from build123d import *

# Parameters (mm, degrees)
MODEL_W                 = 52
MODEL_H                 = 52
MODEL_R                 = 1.5
SALIENTE_EXTRUIR1_DEPTH = 3


with BuildPart() as part:
    # Model → Saliente-Extruir1 (new body)
    with BuildSketch(Plane.XY):
        with Locations((66, 205)):
            Rectangle(MODEL_W, MODEL_H)
        with Locations((51, 190)):
            Circle(MODEL_R, mode=Mode.SUBTRACT)
        with Locations((81, 190)):
            Circle(MODEL_R, mode=Mode.SUBTRACT)
        with Locations((81, 220)):
            Circle(MODEL_R, mode=Mode.SUBTRACT)
        with Locations((51, 220)):
            Circle(MODEL_R, mode=Mode.SUBTRACT)
        Polygon((56, 226), (56, 215), (46, 215), (46, 195), (56, 195), (56, 184), (69.4, 184), (69.4, 226), align=None, mode=Mode.SUBTRACT)
        Polygon((72.4, 226), (72.4, 184), (76, 184), (76, 195), (85, 195), (85, 215), (76, 215), (76, 226), align=None, mode=Mode.SUBTRACT)
    extrude(amount=SALIENTE_EXTRUIR1_DEPTH)


solid = part.part
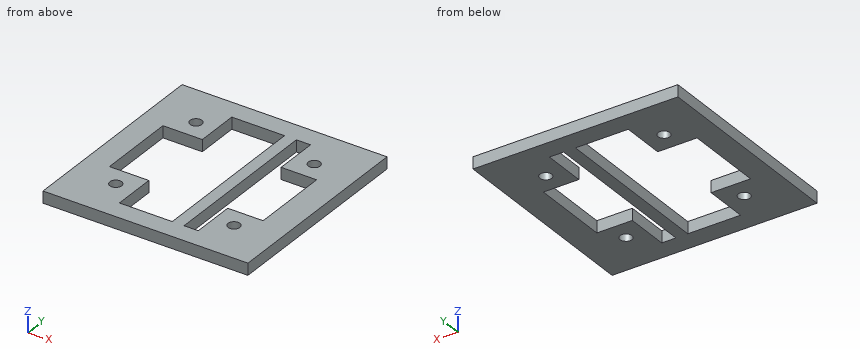
Geometry: final body of the model. Coordinates: model frame, mm. Coordinates: 2 decimals unless noted, no trailing zeros. Loops run counter-clockwise (first coordinate to the right, second up) from the corner with the lowest first, then second, coordinate; pieces in that order, holes last. Notation, with made-up numbers: M 65.5,21.5 L 117.5,21.5 A22 cw 117.5,51.5 Z; hole C 76,2.5 d11. An arc over 180 degrees is marked long. One line per item, written item: value. Start each with the question number.
1) Pin query (flat end, axial travel): P1, Ø12, axis at x = 63.5, y = 201, coming from the +Z side. Return the tip coordinate at first contact, or that it passes through.
2) Cut plane B-B (x = 51). Return loops of the section in (y, z), then the cut area to 3 significant figures.
3) Cut plane D-D (x = 77). Return loops of the section in (y, z), then the cut area to 3 significant figures.
4) Cut plane C-C (y = 190). Return loops of the section in (x, z).
5) Material intervals for L1, parallel to X at y = 213.5, z = 2.45; L2, parallel to Y at x = 51, z = 1.85; L3, parallel to X at y = 190, z = 0.95, sorted ascending. Write a range as from..to.
6) Cut plane A-A (y = 201). Return loops of the section in (x, z), then the cut area to 3 significant figures.
Evaluation:
1. P1: z = 3
2. outline: M 179,0 L 188.5,0 L 188.5,3 L 179,3 Z; M 191.5,0 L 195,0 L 195,3 L 191.5,3 Z; M 215,0 L 218.5,0 L 218.5,3 L 215,3 Z; M 221.5,0 L 231,0 L 231,3 L 221.5,3 Z
2. area: 78.0 mm^2
3. outline: M 179,0 L 195,0 L 195,3 L 179,3 Z; M 215,0 L 231,0 L 231,3 L 215,3 Z
3. area: 96.0 mm^2
4. outline: M 40,0 L 49.5,0 L 49.5,3 L 40,3 Z; M 52.5,0 L 56,0 L 56,3 L 52.5,3 Z; M 69.4,0 L 72.4,0 L 72.4,3 L 69.4,3 Z; M 76,0 L 79.5,0 L 79.5,3 L 76,3 Z; M 82.5,0 L 92,0 L 92,3 L 82.5,3 Z
5. L1: 40..46, 69.4..72.4, 85..92
5. L2: 179..188.5, 191.5..195, 215..218.5, 221.5..231
5. L3: 40..49.5, 52.5..56, 69.4..72.4, 76..79.5, 82.5..92
6. outline: M 40,0 L 46,0 L 46,3 L 40,3 Z; M 69.4,0 L 72.4,0 L 72.4,3 L 69.4,3 Z; M 85,0 L 92,0 L 92,3 L 85,3 Z
6. area: 48.0 mm^2
